Here's the drawing with two shaded views (mm, measured from the low corner). I have some questions. A direction names the side the tool comes from. Coordinates: 2 decimals unless noted, no trailing zeros. Order: outer loops, then holes, each group sorted by start corner. A loop starts at its lowest first (then second) coordinate and runs counter-clockwise, first axis right, second up. Notation, with made-up numbers: (14, 35.5) -> (19, 35.5) arc R19 cw to (19, 39.5) -> close; hole circle Ø4 at (85, -31). An arc over 180 degrees is marked (long way). Write item = value, one per line.
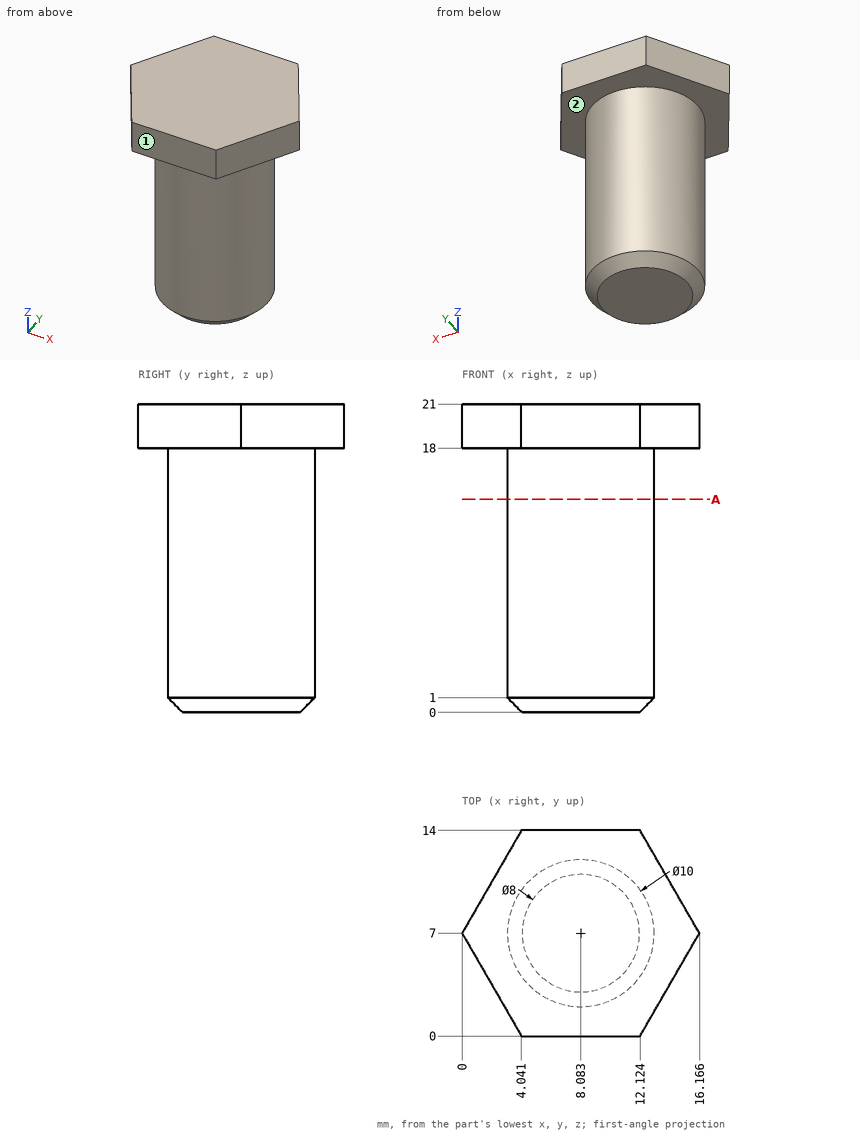
Item 1: I want a section at A-A, the plane z = 14.5. Please give me the cut outline in (x, y).
A:
outline = circle Ø10 at (8.08, 7)
Item 2: For the marked faces 1 and 2, which set-ups out of +Z, -Z, +X, -X, +Y, -Y let a thin tool reach every point of the face, with its end or its side?
A:
face_1 = +Z, -Z, +X, -X, -Y
face_2 = -Z
Item 3: If I drill on probe 1 along Z at (x, y) = (12.5, 13); probe 2 along Y at (x, z) = (11, 15); probe 3 along X at (y, z) = (9.75, 15) (1 decimal), over which ranges is the centre line in solid material (lowest first)?
A:
probe_1 = 18 to 21
probe_2 = 2.94 to 11.06
probe_3 = 3.9 to 12.3
Item 4: I'm going to push flat-ended pins straight in: P1, Ø5, axis at x = 11, y = 2.5, coming from the -Z side; P2, Ø3, axis at x = 12, z = 4.5, coming from the +Y side; P3, Ø6, axis at x = 6.5, z = 6.5, coming from the -Y side; P4, Ø5, axis at x = 4, z = 5, coming from the -Y side. Where does each tip first touch, or does it pass through?
A:
P1 = 0
P2 = 11.38
P3 = 2
P4 = 2.26
